```python
from build123d import *

# Parameters (mm, degrees)
BOSS_EXTRUDE1_DEPTH = 12.7
EXTRUDE_THIN1_START = -6.35
EXTRUDE_THIN1_DEPTH = 12.7
BOSS_EXTRUDE2_DEPTH = 12.7
SKETCH4_W           = 6.35
SKETCH4_H           = 6.35
BOSS_EXTRUDE3_DEPTH = 17.3
FILLET1_R           = 20
CHAMFER1_SIZE       = 10


# Read off the part's stored shape, not the designer's step: Extrude-Thin1
with BuildPart() as part:
    # Sketch1 → Boss-Extrude1 (new body)
    with BuildSketch(Plane(origin=(0, 0, 0), x_dir=(0, 0, -1), z_dir=(1, 0, 0))):
        Polygon((72.847962895, 3.175), (72.847962895, 0), (98.247962895, 0), (98.247962895, 38.1), (91.897962895, 38.1), (91.897962895, 6.35), (79.197962895, 6.35), (79.197962895, 38.1), (72.847962895, 38.1), align=None)
    extrude(amount=BOSS_EXTRUDE1_DEPTH)



with BuildPart() as body_2:
    # Extrude-Thin1 outline → Extrude-Thin1 (new body)
    with BuildSketch(Plane(origin=(6.35, 0, 0), x_dir=(0, 0, -1), z_dir=(1, 0, 0)).offset(EXTRUDE_THIN1_START)):
        with BuildLine():
            Line((72.417611424, 0.000950446), (72.262248261, 6.349049554))
            add(Edge.make_bspline(
                [(72.262248261, 6.349049554), (63.021883212, 6.122901173), (54.028914036, 6.667445615), (36.522694485, 9.291097632), (28.009187017, 11.370086401), (11.442378767, 17.064926737), (3.388803369, 20.680920683), (-12.273002956, 29.461644656), (-19.881272632, 34.626626552), (-27.26926203, 40.573319228)],
                knots=[0, 0, 0, 0, 0.25, 0.25, 0.5, 0.5, 0.75, 0.75, 1, 1, 1, 1], degree=3))
            Line((-27.26926203, 40.573319228), (-31.250878284, 35.626680772))
            add(Edge.make_bspline(
                [(72.417611424, 0.000950446), (62.82712633, -0.233766762), (53.463624565, 0.331247938), (35.205660639, 3.067563666), (26.31145557, 5.238983498), (9.011597154, 11.185809829), (0.606218421, 14.961073948), (-15.70112511, 24.103715563), (-23.603051159, 29.470841193), (-31.250878284, 35.626680772)],
                knots=[0, 0, 0, 0, 0.25, 0.25, 0.5, 0.5, 0.75, 0.75, 1, 1, 1, 1], degree=3))
        make_face()
    extrude(amount=EXTRUDE_THIN1_DEPTH)


with BuildPart() as part_1:
    add(part.part)

    add(body_2.part)  # Boss-Extrude2 merges body 2
    # Sketch3 → Boss-Extrude2 (add)
    with BuildSketch(Plane(origin=(12.7, 0, 0), x_dir=(0, 0, -1), z_dir=(1, 0, 0))):
        Polygon((72.262248261, 6.349049554), (72.847962895, 6.349049554), (72.847962895, 0), (72.417611424, 0.000950446), align=None)
    extrude(amount=-BOSS_EXTRUDE2_DEPTH)

    # Sketch4 → Boss-Extrude3 (add)
    with BuildSketch(Plane(origin=(12.7, 0, 0), x_dir=(0, 0, -1), z_dir=(1, 0, 0))):
        with Locations((76.022962895, 34.925)):
            Rectangle(SKETCH4_W, SKETCH4_H)
        with Locations((95.072962895, 34.925)):
            Rectangle(SKETCH4_W, SKETCH4_H)
    extrude(amount=BOSS_EXTRUDE3_DEPTH)

    # Fillet1
    fillet1_edges = [part_1.edges().sort_by_distance(p)[0] for p in [
        (6.35, 6.349049554, -72.847962895),
    ]]
    fillet(fillet1_edges, radius=FILLET1_R)

    # Chamfer1
    # the kernel refuses this chamfer: 10 mm, written as the material it adds along each edge
    with BuildSketch(Plane(origin=(0, 6.35, -91.897962895), x_dir=(0, -0.027495876610586664, 0.9996219169112968), z_dir=(1, 0, 0)), Plane(origin=(0, 6.35, -79.197962895), x_dir=(0, 0.9996219169112968, 0.027495876610586317), z_dir=(1, 0, 0))) as chamfer1_piece_1:
        Polygon((CHAMFER1_SIZE * 0.999621916911, -CHAMFER1_SIZE * 0.0274958766106), (-CHAMFER1_SIZE * 0.0274958766106, -CHAMFER1_SIZE * 0.999621916911), (0, 0), align=None)
    extrude(amount=12.7)


solid = part_1.part
```
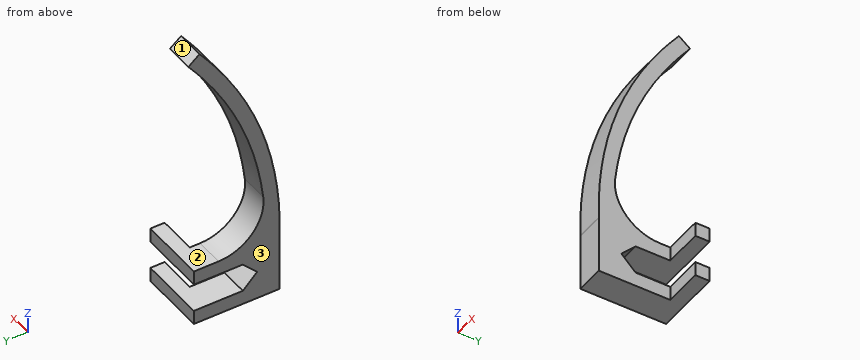
Can you work these out from the model? Positions are in its coordinate system, mm. Face numbers are marked on the shaded views. Round coordinates to 2 decimals unless told otherwise and drop trailing zeros. Loops run counter-clockwise (first coordinate to the right, second up) from the corner with the lowest first, then second, coordinate; pieces in that order, holes last. Notation, with made-up numbers: (48.5, 87) -> (64.5, 87) arc R6 cw to (64.5, 97) -> close; hole circle Ø9 at (80.5, 59). An arc over 180 degrees is marked (long way). One line per item, written item: value. Start each with the question number.
1. If we section it at B-B, the plane y = 25: Give the number of separate pieces and of enclosed holes in the cut face, then the cut area to 3 significant figures.
2. For pin 1 (6 mm diameter, centred on y = 14.5, z = 4, fed in from +X); pin 2 (1.9 mm diameter, centred on x = 24.5, z = -75, fed in from -Y); pin 3 (4 mm diameter, centred on x = 4.5, z = -50, fed in from +Y); pin 4 (2 mm diameter, centred on x = 17.5, y = 30, fed in from -Z), each with a flat end and sliding along its axis, tell me the tip position at first contact or that it passes through.
3. If I drill on probe 1 along Z at (x, y) = (13.5, 32.5); probe 2 along X at (y, z) = (16, -69.5); probe 3 along Z at (x, y) = (10, 24.5), over which ranges is the centre line in solid material (lowest first)?
4. If we section it at C-C, the plane z = -83: Write out the boundary of the cut face in (x, y).
5. If we section it at A-A, the plane x = 28: Write out the boundary of the cut face in (y, z).
6. If we mould it in two halves opening along Z, with no side actions, what happens to the marked faces 1, 2 and 3? For each: pulls with the +Z half, pulls with the -Z half, needs draft (parallel to the pull), parting line crosses it, or undercut.
Calculated:
1. separate pieces: 3
1. enclosed holes: 0
1. area: 319 mm²
2. pin 1: stops at x = 12.7
2. pin 2: stops at y = 31.75
2. pin 3: stops at y = 7.6
2. pin 4: passes through
3. probe 1: z = -98.25 to -91.9, -79.2 to -72.85
3. probe 2: x = 0 to 12.7
3. probe 3: z = -98.25 to -91.9, -79.2 to -72.67, 3.41 to 15.82
4. outline: (0, 0) -> (12.7, 0) -> (12.7, 12.55) -> (0, 12.55) -> close
5. outline: (31.75, -98.25) -> (38.1, -98.25) -> (38.1, -91.9) -> (31.75, -91.9) -> close; (31.75, -79.2) -> (38.1, -79.2) -> (38.1, -72.85) -> (31.75, -72.85) -> close
6. face 1: pulls with the +Z half
6. face 2: undercut
6. face 3: needs draft
